```python
from build123d import *

# Parameters (mm, degrees)
SKETCH1_R           = 41.275
BOSS_EXTRUDE1_DEPTH = 22.86
CUT_EXTRUDE1_REACH  = 64.688
SKETCH2_R           = 2.5
FILLET2_R           = 10


with BuildPart() as part:
    # Sketch1 → Boss-Extrude1 (new body)
    with BuildSketch(Plane.XY):
        Circle(SKETCH1_R)
    extrude(amount=BOSS_EXTRUDE1_DEPTH)

    # Sketch2 → Cut-Extrude1 (cut, up to next)
    with BuildSketch(Plane.XY, mode=Mode.PRIVATE) as cut_extrude1_sk1:
        with Locations(Location((0, 0, 0), (0, 0, 180))):
            Circle(SKETCH2_R)
    cut_extrude1_tool1 = extrude(cut_extrude1_sk1.sketch, amount=CUT_EXTRUDE1_REACH, mode=Mode.PRIVATE) & part.part
    add(cut_extrude1_tool1.solids().sort_by_distance((0, 0, 0))[0], mode=Mode.SUBTRACT)

    # Fillet2
    fillet2_edges = [part.edges().sort_by_distance(p)[0] for p in [
        (-41.275, 0, 0),
        (-41.275, 0, 22.86),
    ]]
    fillet(fillet2_edges, radius=FILLET2_R)


solid = part.part
```
For this review, take the finished solid that the model builds, in its own axes (mm). Coordinates: 2 decimals unless noted, no trailing zeros. Write each loop counter-clockwise with the first axis right and the second up, starting at its lowest first coordinate (ties: lowest second). Pieces come first, ordered by that corner, then holes.
(1) Add section D-D on z = 21. Give the boundary of the cut face in (x, y).
(2) Add section A-A on x = 0. Give the boundary of the cut face in (y, z) (3 decimals).
(3) Wall thickness on probe 1 along Y at (x, z) = (0, 11.75) (3 decimals); probe 2 along Y at (x, z) = (0, 14); probe 3 along X at (y, z) = (19.5, 2.5): over which ranges is each line inside the solid? List them lowest first.
(4) The part is to be moulded in two halves that separate along X. For faces 1 (the face through (2.5, -0.1, 11.3)), 2 (the face through (-8.948, -40.293, 11.41)), 3 (the face through (0, -7, 0)), say which applies: +X half, -X half, draft (parallel to the pull), parting line (faces both ways), or undercut.
(5) Add section C-C on z = 4.75. Give the boundary of the cut face in (x, y), then the cut area to 3 significant figures.
(6) For pin 1 Ø12 at (x, y) = (7.5, -32) entering from +Z; pin 2 Ø3 at (y, z) = (-15, 11) entering from -X; pin 3 Ø1 at (x, z) = (23.5, 7) entering from -Y; pin 4 Ø1.5 at (y, z) = (1, 10) entering from -X, all flat-tipped, find the tip position at first contact; note any pin that passes through.
Answer sheet:
1. outline: circle Ø74.17 at (0, 0); hole circle Ø5 at (0, 0)
2. outline: (-41.275, 10) arc R10 ccw to (-31.275, 0) - (-2.5, 0) - (-2.5, 22.86) - (-31.275, 22.86) arc R10 ccw to (-41.275, 12.86) - close; (2.5, 0) - (31.275, 0) arc R10 ccw to (41.275, 10) - (41.275, 12.86) arc R10 ccw to (31.275, 22.86) - (2.5, 22.86) - close
3. probe 1: y = -41.275 to -2.5, 2.5 to 41.275
3. probe 2: y = -41.21 to -2.5, 2.5 to 41.21
3. probe 3: x = -32.49 to 32.49
4. face 1: undercut
4. face 2: parting line
4. face 3: draft
5. outline: circle Ø79.57 at (0, 0); hole circle Ø5 at (0, 0)
5. area: 4,950 mm2
6. pin 1: stops at z = 22.86
6. pin 2: stops at x = -39
6. pin 3: stops at y = -33.76
6. pin 4: stops at x = -41.27
